Here's the drawing with two shaded views (mm, measured from the low corner). I have some questions. Coordinates: 2 decimals unless noted, no trailing zeros. Write each loop counter-clockwise with the first axis right and the second up, starting at its lowest first coordinate (ties: lowest second). Pieces come first, ordered by that corner, then holes.
Item 1: I'm going to push flat-ended pins straight in: pin 1 Ø5.5 at (y, z) = (6, 10) entering from -X; pin 2 Ø12.5 at (x, y) = (163, 137.5) entering from +Z (1 decimal); pin 3 Ø5.5 at (x, z) = (10.5, 7) entering from -Y. Where does each tip first touch, or does it pass through?
Item 2: If I drill on line 1 (X direction, y = 76, z = 13.5); line 2 (Y direction, x = 78, z = 14.25), over which ranges is the centre line in solid material (lowest first)?
Item 3: If we section it at B-B (y = 45): Please give me the cut outline in (x, z).
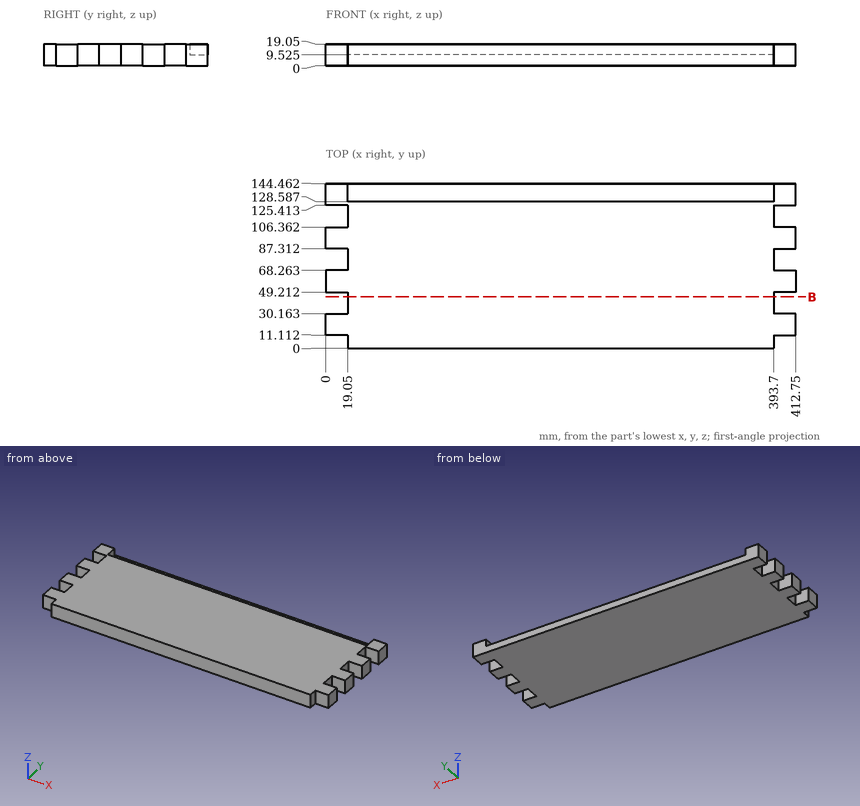
Answer list:
1. pin 1: stops at x = 19.05
1. pin 2: stops at z = 9.5
1. pin 3: stops at y = 11.11
2. line 1: x = 19.05 to 393.7
2. line 2: y = 0 to 128.59
3. outline: (19.05, 0) - (393.7, 0) - (393.7, 19.05) - (19.05, 19.05) - close
